Here's how the part is built. I have some questions about the finished solid (model axes, mm). Give positions to 0.01 mm unless a question says otherwise; leave off trailing zeros. Loops run counter-clockwise (first coordinate to the right, second up) from the corner with the lowest first, then second, coordinate; pieces in that order, holes last.
Q1. I need wall thicknesses on line 1 (X direction, y = -1, z = 1.95); line 2 (X direction, y = 12.5, z = 0.2); line 3 (Y direction, x = 11.5, z = 1.25). Which ranges of each line are inside material? Lowest first, please.
Q2. If we section it at A-A (y = 0): Please give me the cut outline in (x, z).
Q3. Will these pins go through, and if not, where does the flat tip stop? P1, Ø4, axis at x = -10.25, y = -10.25, coming from the +Z side; P2, Ø6.5, axis at x = 14.5, y = 0, coming from the -Z side; P3, Ø1, axis at y = -11, z = 1, coming from the -X side.
Q4. If we section it at D-D (z = 0.55): Give the number of separate pieces and of enclosed holes in the cut face, plus the area to 3 significant figures.
Q5. If we section it at B-B (x = 0): Please give me the cut outline in (y, z).
Q6. If we section it at C-C (y = -11.5): Please give me the cut outline in (x, z), plus the area to 3 significant figures.
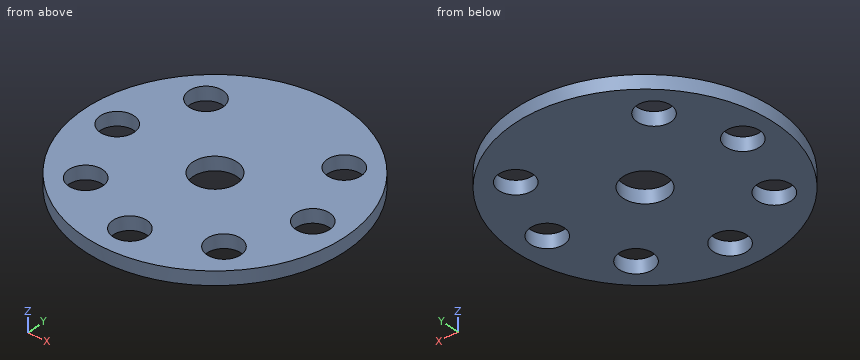
from build123d import *

# Parameters (mm, degrees)
SKETCH_1_R          = 19.25
EXTRUDE_1_DEPTH     = 2
SKETCH_4_R          = 2.5
SKETCH_4_R_2        = 3.25
CUT_EXTRUDE_2_DEPTH = 3


with BuildPart() as part:
    # Эскиз1 → Вытянуть1 (new body)
    with BuildSketch(Plane.XY):
        Circle(SKETCH_1_R)
    extrude(amount=EXTRUDE_1_DEPTH)

    # Эскиз4 → Вытянуть2 (cut, through all)
    with BuildSketch(Plane.XY.offset(2)):
        with Locations((-10.253048327, 10.253048327)):
            Circle(SKETCH_4_R)
        with Locations((-14.5, 0)):
            Circle(SKETCH_4_R)
        with Locations((-10.253048327, -10.253048327)):
            Circle(SKETCH_4_R)
        with Locations((0, -14.5)):
            Circle(SKETCH_4_R)
        with Locations((10.253048327, -10.253048327)):
            Circle(SKETCH_4_R)
        with Locations((14.5, 0)):
            Circle(SKETCH_4_R)
        with Locations((10.253048327, 10.253048327)):
            Circle(SKETCH_4_R)
        Circle(SKETCH_4_R_2)
    extrude(amount=-CUT_EXTRUDE_2_DEPTH, mode=Mode.SUBTRACT)


solid = part.part
Check sheet entries:
1. line 1: x = -19.22 to -16.79, -12.21 to -3.09, 3.09 to 12.21, 16.79 to 19.22
1. line 2: x = -14.64 to -11.35, -9.16 to 9.16, 11.35 to 14.64
1. line 3: y = -15.44 to -12.42, -8.09 to 8.09, 12.42 to 15.44
2. outline: (-19.25, 0) - (-17, 0) - (-17, 2) - (-19.25, 2) - close; (-12, 0) - (-3.25, 0) - (-3.25, 2) - (-12, 2) - close; (3.25, 0) - (12, 0) - (12, 2) - (3.25, 2) - close; (17, 0) - (19.25, 0) - (19.25, 2) - (17, 2) - close
3. P1: passes through
3. P2: stops at z = 0
3. P3: stops at x = -16.13
4. separate pieces: 1
4. enclosed holes: 8
4. area: 994 mm2
5. outline: (-19.25, 0) - (-17, 0) - (-17, 2) - (-19.25, 2) - close; (-12, 0) - (-3.25, 0) - (-3.25, 2) - (-12, 2) - close; (3.25, 0) - (19.25, 0) - (19.25, 2) - (3.25, 2) - close
6. outline: (-15.44, 0) - (-12.42, 0) - (-12.42, 2) - (-15.44, 2) - close; (-8.09, 0) - (8.09, 0) - (8.09, 2) - (-8.09, 2) - close; (12.42, 0) - (15.44, 0) - (15.44, 2) - (12.42, 2) - close
6. area: 44.4 mm2
